Input: part model. Units: mm. Frame: model coordinates. Face numbers are marked on the shaded views. A direction names the side the tool comes from. Coordinates: 2 decimals unless noted, no trailing zeros. Write each loop counter-clockwise with the first axis right and the second up, starting at its lowest first coordinate (ties: lowest second). Pieces come first, ordered by that corner, then holes. Notation, with made-up numbers: (81, 65.25) - (97, 65.25) arc R19 ccw to (97, 79.25) - close; hole circle Ø8 at (-28, 72.25). An arc over 180 degrees is marked (long way). Put each result on its own line as item: value. Start each with the question number.
1. Cut plane A-A, the plane z = 0. Return loops of the section in (x, y).
2. Cut plane B-B, the plane y = 0. Return loops of the section in (x, z), and give its area (3 significant figures).
3. Access query for the marked faces 1, 2 and 3. Directions: +Z, -Z, +X, -X, +Y, -Y. A direction counts if a zero-diameter tool reaches every point of the face in a straight line with its end or side. Return the directions, or none.
4. Line query: line 1 (X direction, y = 6.75, z = -5); line 2 (X direction, y = -6.75, z = -2.75); line 3 (Z direction, x = 40.5, y = 3.5). Output: solid intervals per line, ascending.
5. Cut plane D-D, the plane y = -6.25. Return loops of the section in (x, z), and give its area (3 significant figures).
6. Cut plane C-C, the plane x = 14. Return loops of the section in (y, z).
7. Pin query (flat end, axial travel): pin 1 (2 mm diameter, centred on x = 36.5, z = 6.5, fed in from +Y); pin 2 (8 mm diameter, centred on y = 0, z = -5.5, fed in from +X); pin 3 (1 mm diameter, centred on x = 24.5, z = 9.5, fed in from +Y); pin 4 (1.5 mm diameter, centred on x = 25, y = 0, fed in from +Z). Return the tip coordinate at first contact, or that it passes through.
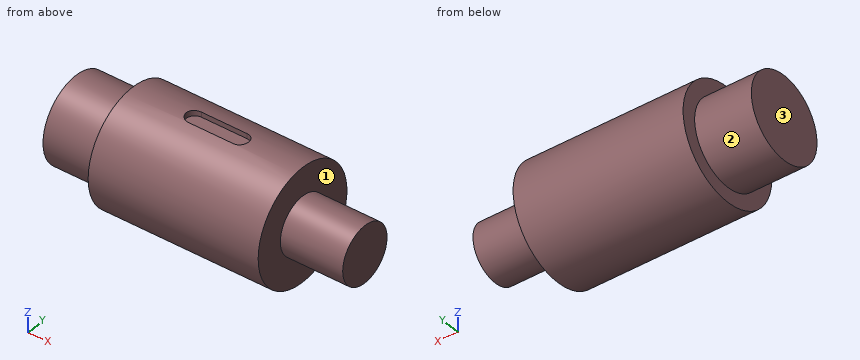
from build123d import *

# Parameters (mm, degrees)
CUT_EXTRUDE1_START = 9
CUT_EXTRUDE1_DEPTH = 10


with BuildPart() as part:
    # Sketch1 → Revolve1 (revolve)
    with BuildSketch(Plane.XY, mode=Mode.PRIVATE) as revolve1_sk:
        Polygon((0, 0), (0, 7.4), (10, 7.4), (10, 10), (40, 10), (40, 5), (51, 5), (51, 0), align=None)
    revolve(revolve1_sk.sketch.rotate(Axis((0, 0, 0), (1, 0, 0)), 180), axis=Axis((0, 0, 0), (1, 0, 0)))

    # Sketch2 → Cut-Extrude1 (cut)
    with BuildSketch(Plane.XY.offset(CUT_EXTRUDE1_START)):
        with BuildLine():
            Line((21, 1.5), (29, 1.5))
            ThreePointArc((29, 1.5), (30.5, 0), (29, -1.5))
            Line((29, -1.5), (21, -1.5))
            ThreePointArc((21, -1.5), (19.5, 0), (21, 1.5))
        make_face()
    extrude(amount=CUT_EXTRUDE1_DEPTH, mode=Mode.SUBTRACT)


solid = part.part
Report:
1. outline: (0, -7.4) - (10, -7.4) - (10, -10) - (40, -10) - (40, -5) - (51, -5) - (51, 5) - (40, 5) - (40, 10) - (10, 10) - (10, 7.4) - (0, 7.4) - close
2. outline: (0, -7.4) - (10, -7.4) - (10, -10) - (40, -10) - (40, -5) - (51, -5) - (51, 5) - (40, 5) - (40, 10) - (30.5, 10) - (30.5, 9) - (19.5, 9) - (19.5, 10) - (10, 10) - (10, 7.4) - (0, 7.4) - close
2. area: 847 mm^2
3. face 1: +X
3. face 2: -X
3. face 3: +Z, -Z, -X, +Y, -Y
4. line 1: x = 10 to 40
4. line 2: x = 0 to 40
4. line 3: z = -3.57 to 3.57
5. outline: (0, -3.96) - (10, -3.96) - (10, -7.81) - (40, -7.81) - (40, 7.81) - (10, 7.81) - (10, 3.96) - (0, 3.96) - close
5. area: 548 mm^2
6. outline: circle Ø20 at (0, 0)
7. pin 1: stops at y = 8.35
7. pin 2: stops at x = 51
7. pin 3: stops at y = 4.36
7. pin 4: stops at z = 9
